Could you check a few things on this model? Use its own coordinates, in mm. Face numbers are marked on the shaded views. A direction names the side the tool comes from. Give positions to 0.01 mm unless a question says otherwise; leave off trailing zeros. Order: outer loops, then holes, each group sorted by start corner. A loop starts at its lowest first (then second) coordinate and runs counter-clockwise, first axis right, second up.
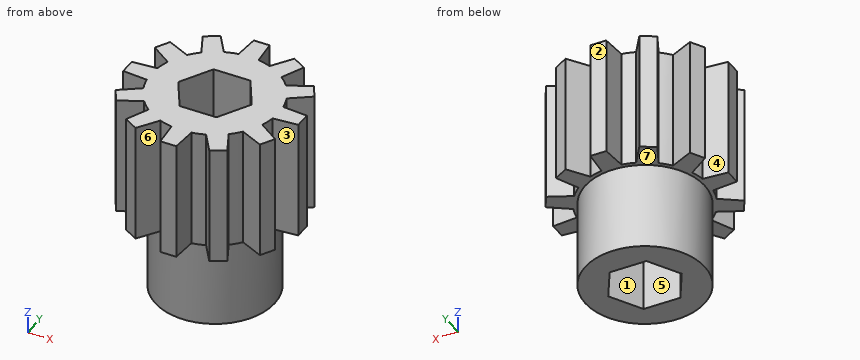
Autodesk Inventor part; units mm, degrees
ref_plane "YZ Plane" through (0, 0, 0) normal (1, 0, 0) x (0, 1, 0)
ref_plane "XZ Plane" through (0, 0, 0) normal (0, 1, 0) x (-1, 0, 0)
ref_plane "XY Plane" through (0, 0, 0) normal (0, 0, 1) x (1, 0, 0)
sketch "Sketch1" plane through (0, 0, 0) normal (0, 0, 1) x (1, 0, 0)
  circle A0 centre (0, 0) radius 11.9062
  dimension "d0" = 23.8125
extrude "Extrusion1" add sketch "Sketch1" along normal blind 41.275
sketch "Sketch2" plane through (0, 0, 41.275) normal (0, 0, 1) x (1, 0, 0)
  circle A0 centre (0, 0) radius 12.7
  dimension "d3" = 25.4
extrude "Extrusion2" add sketch "Sketch2" against normal blind 23.8125
sketch "Sketch3" plane through (0, 0, 41.275) normal (0, 0, 1) x (1, 0, 0)
  line L0 (-3.6662, 6.35) -> (3.6662, 6.35)
  line L1 (3.6662, 6.35) -> (7.3323, 0)
  line L2 (7.3323, 0) -> (3.6662, -6.35)
  line L3 (3.6662, -6.35) -> (-3.6662, -6.35)
  line L4 (-3.6662, -6.35) -> (-7.3323, 0)
  line L5 (-7.3323, 0) -> (-3.6662, 6.35)
  point P0 (0, 0)
  dimension "d6" = 12.7
  dimension "d7" = 12.7
  dimension "d8" = 12.7
  dimension "d9" = 120
  dimension "d10" = 120
  dimension "d11" = 6.35
  dimension "d12" = 6.35
  dimension "d13" = 6.35
extrude "Extrusion3" cut sketch "Sketch3" against normal blind 50.8
sketch "Sketch4" plane through (0, 0, 41.275) normal (0, 0, 1) x (1, 0, 0)
  line L0 (-7.3323, 0) -> (-3.6662, 6.35)
  line L1 (-3.6662, 6.35) -> (3.6662, 6.35)
  line L2 (3.6662, 6.35) -> (7.3323, 0)
  line L3 (7.3323, 0) -> (3.6662, -6.35)
  line L4 (3.6662, -6.35) -> (-3.6662, -6.35)
  line L5 (-3.6662, -6.35) -> (-7.3323, 0)
  circle A0 centre (0, 0) radius 12.7
  line L6 (0, 12.7) -> (0, 17.4625) construction
  line L7 (0, 12.7) -> (4.7625, 12.7) construction
  line L8 (0, 0) -> (1.9867, 12.5436) construction
  circle A1 centre (0, 0) radius 12.7 construction
  line L9 (0, 0) -> (12.7, 0) construction
  line L10 (0, 0) -> (-1.9867, 12.5436) construction
  line L11 (0, 0) -> (12.7, 0) construction
  line L12 (0, 17.4625) -> (0.7937, 17.4625) construction
  line L13 (0, 17.4625) -> (0.7937, 17.4625) construction
  line L14 (0, 17.4625) -> (-1.5875, 17.4625) construction
  line L15 (0, 17.4625) -> (1.5875, 17.4625) construction
  line L16 (-1.9867, 12.5436) -> (-1.5875, 17.4625)
  line L17 (-1.5875, 17.4625) -> (1.5875, 17.4625)
  line L18 (1.5875, 17.4625) -> (1.9867, 12.5436)
  line L19 (-1.9867, 12.5436) -> (1.9867, 12.5436)
  line L20 (-6.35, 10.9985) -> (-8.7312, 15.123) construction
  line L21 (-6.35, 10.9985) -> (-2.2256, 13.3798) construction
  line L22 (0, 0) -> (-4.5513, 11.8565) construction
  line L23 (0, 0) -> (-7.9924, 9.8698) construction
  line L24 (-8.7312, 15.123) -> (-8.0438, 15.5198) construction
  line L25 (-8.7312, 15.123) -> (-8.0438, 15.5198) construction
  line L26 (-8.7312, 15.123) -> (-10.1061, 14.3292) construction
  line L27 (-8.7312, 15.123) -> (-7.3564, 15.9167) construction
  line L28 (-7.9924, 9.8698) -> (-10.1061, 14.3292)
  line L29 (-10.1061, 14.3292) -> (-7.3564, 15.9167)
  line L30 (-7.3564, 15.9167) -> (-4.5513, 11.8565)
  line L31 (-7.9924, 9.8698) -> (-4.5513, 11.8565)
  line L32 (-10.9985, 6.35) -> (-15.123, 8.7313) construction
  line L33 (-10.9985, 6.35) -> (-8.6173, 10.4744) construction
  line L34 (0, 0) -> (-9.8698, 7.9924) construction
  line L35 (0, 0) -> (-11.8565, 4.5513) construction
  line L36 (-15.123, 8.7313) -> (-14.7261, 9.4187) construction
  line L37 (-15.123, 8.7313) -> (-14.7261, 9.4187) construction
  line L38 (-15.123, 8.7313) -> (-15.9167, 7.3564) construction
  line L39 (-15.123, 8.7313) -> (-14.3292, 10.1061) construction
  line L40 (-11.8565, 4.5513) -> (-15.9167, 7.3564)
  line L41 (-15.9167, 7.3564) -> (-14.3292, 10.1061)
  line L42 (-14.3292, 10.1061) -> (-9.8698, 7.9924)
  line L43 (-11.8565, 4.5513) -> (-9.8698, 7.9924)
  line L44 (-12.7, 0) -> (-17.4625, 0) construction
  line L45 (-12.7, 0) -> (-12.7, 4.7625) construction
  line L46 (0, 0) -> (-12.5436, 1.9867) construction
  line L47 (0, 0) -> (-12.5436, -1.9867) construction
  line L48 (-17.4625, 0) -> (-17.4625, 0.7938) construction
  line L49 (-17.4625, 0) -> (-17.4625, 0.7938) construction
  line L50 (-17.4625, 0) -> (-17.4625, -1.5875) construction
  line L51 (-17.4625, 0) -> (-17.4625, 1.5875) construction
  line L52 (-12.5436, -1.9867) -> (-17.4625, -1.5875)
  line L53 (-17.4625, -1.5875) -> (-17.4625, 1.5875)
  line L54 (-17.4625, 1.5875) -> (-12.5436, 1.9867)
  line L55 (-12.5436, -1.9867) -> (-12.5436, 1.9867)
  line L56 (-10.9985, -6.35) -> (-15.123, -8.7312) construction
  line L57 (-10.9985, -6.35) -> (-13.3798, -2.2256) construction
  line L58 (0, 0) -> (-11.8565, -4.5513) construction
  line L59 (0, 0) -> (-9.8698, -7.9924) construction
  line L60 (-15.123, -8.7312) -> (-15.5198, -8.0438) construction
  line L61 (-15.123, -8.7312) -> (-15.5198, -8.0438) construction
  line L62 (-15.123, -8.7312) -> (-14.3292, -10.1061) construction
  line L63 (-15.123, -8.7312) -> (-15.9167, -7.3564) construction
  line L64 (-9.8698, -7.9924) -> (-14.3292, -10.1061)
  line L65 (-14.3292, -10.1061) -> (-15.9167, -7.3564)
  line L66 (-15.9167, -7.3564) -> (-11.8565, -4.5513)
  line L67 (-9.8698, -7.9924) -> (-11.8565, -4.5513)
  line L68 (-6.35, -10.9985) -> (-8.7313, -15.123) construction
  line L69 (-6.35, -10.9985) -> (-10.4744, -8.6173) construction
  line L70 (0, 0) -> (-7.9924, -9.8698) construction
  line L71 (0, 0) -> (-4.5513, -11.8565) construction
  line L72 (-8.7313, -15.123) -> (-9.4187, -14.7261) construction
  line L73 (-8.7313, -15.123) -> (-9.4187, -14.7261) construction
  line L74 (-8.7313, -15.123) -> (-7.3564, -15.9167) construction
  line L75 (-8.7313, -15.123) -> (-10.1061, -14.3292) construction
  line L76 (-4.5513, -11.8565) -> (-7.3564, -15.9167)
  line L77 (-7.3564, -15.9167) -> (-10.1061, -14.3292)
  line L78 (-10.1061, -14.3292) -> (-7.9924, -9.8698)
  line L79 (-4.5513, -11.8565) -> (-7.9924, -9.8698)
  line L80 (0, -12.7) -> (0, -17.4625) construction
  line L81 (0, -12.7) -> (-4.7625, -12.7) construction
  line L82 (0, 0) -> (-1.9867, -12.5436) construction
  line L83 (0, 0) -> (1.9867, -12.5436) construction
  line L84 (0, -17.4625) -> (-0.7938, -17.4625) construction
  line L85 (0, -17.4625) -> (-0.7938, -17.4625) construction
  line L86 (0, -17.4625) -> (1.5875, -17.4625) construction
  line L87 (0, -17.4625) -> (-1.5875, -17.4625) construction
  line L88 (1.9867, -12.5436) -> (1.5875, -17.4625)
  line L89 (1.5875, -17.4625) -> (-1.5875, -17.4625)
  line L90 (-1.5875, -17.4625) -> (-1.9867, -12.5436)
  line L91 (1.9867, -12.5436) -> (-1.9867, -12.5436)
  line L92 (6.35, -10.9985) -> (8.7312, -15.123) construction
  line L93 (6.35, -10.9985) -> (2.2256, -13.3798) construction
  line L94 (0, 0) -> (4.5513, -11.8565) construction
  line L95 (0, 0) -> (7.9924, -9.8698) construction
  line L96 (8.7312, -15.123) -> (8.0438, -15.5198) construction
  line L97 (8.7312, -15.123) -> (8.0438, -15.5198) construction
  line L98 (8.7312, -15.123) -> (10.1061, -14.3292) construction
  line L99 (8.7312, -15.123) -> (7.3564, -15.9167) construction
  line L100 (7.9924, -9.8698) -> (10.1061, -14.3292)
  line L101 (10.1061, -14.3292) -> (7.3564, -15.9167)
  line L102 (7.3564, -15.9167) -> (4.5513, -11.8565)
  line L103 (7.9924, -9.8698) -> (4.5513, -11.8565)
  line L104 (10.9985, -6.35) -> (15.123, -8.7313) construction
  line L105 (10.9985, -6.35) -> (8.6173, -10.4744) construction
  line L106 (0, 0) -> (9.8698, -7.9924) construction
  line L107 (0, 0) -> (11.8565, -4.5513) construction
  line L108 (15.123, -8.7313) -> (14.7261, -9.4187) construction
  line L109 (15.123, -8.7313) -> (14.7261, -9.4187) construction
  line L110 (15.123, -8.7313) -> (15.9167, -7.3564) construction
  line L111 (15.123, -8.7313) -> (14.3292, -10.1061) construction
  line L112 (11.8565, -4.5513) -> (15.9167, -7.3564)
  line L113 (15.9167, -7.3564) -> (14.3292, -10.1061)
  line L114 (14.3292, -10.1061) -> (9.8698, -7.9924)
  line L115 (11.8565, -4.5513) -> (9.8698, -7.9924)
  line L116 (12.7, 0) -> (17.4625, 0) construction
  line L117 (12.7, 0) -> (12.7, -4.7625) construction
  line L118 (0, 0) -> (12.5436, -1.9867) construction
  line L119 (0, 0) -> (12.5436, 1.9867) construction
  line L120 (17.4625, 0) -> (17.4625, -0.7938) construction
  line L121 (17.4625, 0) -> (17.4625, -0.7938) construction
  line L122 (17.4625, 0) -> (17.4625, 1.5875) construction
  line L123 (17.4625, 0) -> (17.4625, -1.5875) construction
  line L124 (12.5436, 1.9867) -> (17.4625, 1.5875)
  line L125 (17.4625, 1.5875) -> (17.4625, -1.5875)
  line L126 (17.4625, -1.5875) -> (12.5436, -1.9867)
  line L127 (12.5436, 1.9867) -> (12.5436, -1.9867)
  line L128 (10.9985, 6.35) -> (15.123, 8.7313) construction
  line L129 (10.9985, 6.35) -> (13.3798, 2.2256) construction
  line L130 (0, 0) -> (11.8565, 4.5513) construction
  line L131 (0, 0) -> (9.8698, 7.9924) construction
  line L132 (15.123, 8.7313) -> (15.5198, 8.0438) construction
  line L133 (15.123, 8.7313) -> (15.5198, 8.0438) construction
  line L134 (15.123, 8.7313) -> (14.3292, 10.1061) construction
  line L135 (15.123, 8.7313) -> (15.9167, 7.3564) construction
  line L136 (9.8698, 7.9924) -> (14.3292, 10.1061)
  line L137 (14.3292, 10.1061) -> (15.9167, 7.3564)
  line L138 (15.9167, 7.3564) -> (11.8565, 4.5513)
  line L139 (9.8698, 7.9924) -> (11.8565, 4.5513)
  line L140 (6.35, 10.9985) -> (8.7312, 15.123) construction
  line L141 (6.35, 10.9985) -> (10.4744, 8.6173) construction
  line L142 (0, 0) -> (7.9924, 9.8698) construction
  line L143 (0, 0) -> (4.5513, 11.8565) construction
  line L144 (8.7312, 15.123) -> (9.4187, 14.7261) construction
  line L145 (8.7312, 15.123) -> (9.4187, 14.7261) construction
  line L146 (8.7312, 15.123) -> (7.3564, 15.9167) construction
  line L147 (8.7312, 15.123) -> (10.1061, 14.3292) construction
  line L148 (4.5513, 11.8565) -> (7.3564, 15.9167)
  line L149 (7.3564, 15.9167) -> (10.1061, 14.3292)
  line L150 (10.1061, 14.3292) -> (7.9924, 9.8698)
  line L151 (4.5513, 11.8565) -> (7.9924, 9.8698)
  dimension "d16" = 12.7
  dimension "d17" = 0
  dimension "d18" = 4.7625
  dimension "d19" = 90
  dimension "d20" = 81
  dimension "d21" = 99
  dimension "d22" = 0.7937
  dimension "d23" = 0
  dimension "d24" = 1.5875
  dimension "d25" = 180
  dimension "d28" = 360
extrude "Extrusion4" add sketch "Sketch4" against normal blind 23.8125 contours A0 L127 | A0 L124 L125 L126 | L139 A0 | A0 L136 L137 L138 | L112 L113 L114 A0 | A0 L115 | L151 A0 | A0 L148 L149 L150 | L100 L101 L102 A0 | A0 L103 | L19 A0 | A0 L16 L17 L18 | L88 L89 L90 A0 | A0 L91 | L31 A0 | A0 L28 L29 L30 | L76 L77 L78 A0 | A0 L79 | L43 A0 | A0 L40 L41 L42 | L64 L65 L66 A0 | A0 L67 | L55 A0 | A0 L52 L53 L54
properties part number "pinion" material "Nylon, molybdenum disulphide"
Item 1: We'd pull the mould along X, two halves only. Please class the marked faces 1, 2, 3 and 4: +X half, -X half, draft (parallel to the pull), parting line (faces both ways), or undercut.
Findings:
face 1: undercut
face 2: draft
face 3: +X half
face 4: -X half
Item 2: Imagine slicing it at A-A on z = 12. List the corners of the cut face in (x, y) for me.
Findings:
outline: circle Ø23.81 at (0, 0); hole (-7.33, 0) - (-3.67, -6.35) - (3.67, -6.35) - (7.33, 0) - (3.67, 6.35) - (-3.67, 6.35) - close
Item 3: Imagine slicing it at C-C on y = 1. List the corners of the cut face in (x, z) for me (1 decimal).
Findings:
outline: (-17.5, 17.5) - (-11.9, 17.5) - (-11.9, 0) - (-6.8, 0) - (-6.8, 41.3) - (-17.5, 41.3) - close; (6.8, 0) - (11.9, 0) - (11.9, 17.5) - (17.5, 17.5) - (17.5, 41.3) - (6.8, 41.3) - close
Item 4: For the marked faces 5, 6 and 7, which set-ups out of +Z, -Z, +X, -X, +Y, -Y let a thin tool reach every point of the face, with its end or its side?
Findings:
face 5: +Z, -Z
face 6: +Z, -Z, -Y
face 7: -Z
Item 5: For pin 1 (3.5 mm diameter, centred on x = -1.5, z = 14.5, fed in from -Y); pin 2 (8 mm diameter, centred on x = 0, z = 17, fed in from +Y); pin 3 (2 mm diameter, centred on y = -4, z = 30.5, fed in from -X); pin 4 (4 mm diameter, centred on x = -11, z = 29, fed in from +Y), each with a flat end and sliding along its axis, tell me the tip position at first contact or that it passes through.
Findings:
pin 1: stops at y = -11.91
pin 2: stops at y = 17.46
pin 3: stops at x = -12.51
pin 4: stops at y = 14.97
Item 6: Please list where these lines run through material, in increasing order: line 1 along Y through (x, z) = (14, 26); line 2 along Y through (x, z) = (-9.5, 20.5); line 3 along Z through (x, y) = (-9.5, -14) (1 decimal).
Findings:
line 1: y = -9.95 to -6.03, -1.87 to 1.87, 6.03 to 9.95
line 2: y = -14.68 to -13.05, -8.43 to 8.43, 13.05 to 14.68
line 3: z = 17.5 to 41.3
